```python
from build123d import *

# Parameters (mm, degrees)
SKETCH_1_R      = 40
SKETCH_1_R_2    = 30
EXTRUDE_1_DEPTH = 43
SKETCH_2_R      = 40
EXTRUDE_2_DEPTH = 65
SKETCH_3_R      = 31.5
SKETCH_3_R_2    = 30.5
EXTRUDE_3_DEPTH = 162
FILLET_1_R      = 20
FILLET_2_R      = 20
SKETCH_4_R      = 31.5
SKETCH_4_R_2    = 16
EXTRUDE_4_DEPTH = 1
FILLET_3_R      = 3


with BuildPart() as part:
    # Эскиз1 → Вытянуть1 (new body)
    with BuildSketch(Plane(origin=(0, 0, 0), x_dir=(1, 0, 0), z_dir=(0, 1, 0))):
        with Locations(Location((0, 0, 0), (0, 0, 270))):
            Circle(SKETCH_1_R)
        with Locations(Location((0, 0, 0), (0, 0, 270))):
            Circle(SKETCH_1_R_2, mode=Mode.SUBTRACT)
    extrude(amount=EXTRUDE_1_DEPTH)

    # Эскиз2 → Вытянуть2 (add)
    with BuildSketch(Plane(origin=(0, 43, 0), x_dir=(1, 0, 0), z_dir=(0, 1, 0))):
        with Locations(Location((0, 0, 0), (0, 0, 270))):
            Circle(SKETCH_2_R)
    extrude(amount=EXTRUDE_2_DEPTH)

    # Эскиз3 → Вытянуть3 (add)
    with BuildSketch(Plane(origin=(0, 108, 0), x_dir=(-1, 0, 0), z_dir=(0, 1, 0))):
        with Locations(Location((0, 0, 0), (0, 0, 90))):
            Circle(SKETCH_3_R)
        with Locations(Location((0, 0, 0), (0, 0, 90))):
            Circle(SKETCH_3_R_2, mode=Mode.SUBTRACT)
    extrude(amount=EXTRUDE_3_DEPTH)

    # Скругление1
    # the kernel refuses this fillet: 20 mm, written as the material it adds along each edge
    with BuildSketch(Plane(origin=(0, 108, 0), x_dir=(0, 0, 1), z_dir=(-1, 0, 0))) as fillet_1_piece_1:
        with BuildLine():
            CenterArc((51.5, 16.363068172), FILLET_1_R, 180, 54.900367805)
            Line((31.5, 16.363068172), (31.1, 16.363068172))
            Line((31.1, 16.363068172), (31.1, 0))
            Line((31.1, 0), (31.5, -0.4))
            ThreePointArc((31.5, -0.4), (35.75, -0.4), (39.77, -0.327261363))
            Line((39.77, -0.327261363), (40, 0))
        make_face()
    revolve(axis=Axis((0, 108, 0), (0, 1, 0)))

    # Скругление2
    fillet_2_edges = [part.edges().sort_by_distance(p)[0] for p in [
        (0, 108, -40),
    ]]
    fillet(fillet_2_edges, radius=FILLET_2_R)

    # Эскиз4 → Вытянуть4 (add)
    with BuildSketch(Plane(origin=(0, 270, 0), x_dir=(-1, 0, 0), z_dir=(0, 1, 0))):
        with Locations(Location((0, 0, 0), (0, 0, 270))):
            Circle(SKETCH_4_R)
        with Locations(Location((0, 0, 0), (0, 0, 90))):
            Circle(SKETCH_4_R_2, mode=Mode.SUBTRACT)
    extrude(amount=EXTRUDE_4_DEPTH)

    # Скругление3
    fillet_3_edges = [part.edges().sort_by_distance(p)[0] for p in [
        (0, 271, 31.5),
    ]]
    fillet(fillet_3_edges, radius=FILLET_3_R)


solid = part.part
```
Part model, mm, in its own coordinate system. A direction names the side the tool comes from. Coordinates: 2 decimals unless noted, no trailing zeros. Write each loop counter-clockwise with the first axis right and the second up, starting at its lowest first coordinate (ties: lowest second). Pieces come first, ordered by that corner, then holes.
Item 1: Slice it at B-B (y = 21). Write the cut outline in (x, z).
Item 2: Pin check, flat tips, straight feed: pin 1 (5 mm diameter, centred on x = 30.5, y = 157.5, fed in from -Z); pin 2 (5 mm diameter, centred on y = 67, z = -19.5, fed in from -X); pin 3 (4 mm diameter, centred on y = 216, z = -11, fed in from -X). Stop position of each tip, or through.
Item 3: Slice it at A-A (y = 247). Write the cut outline in (x, z).
Item 4: Probe line 1 (Y direction, x = -12.5, z = -16); line 2 (X direction, y = 28, z = 0); line 3 (X direction, y = 169, z = -1.5). List the from-to ranges inside material, lowest first.
Item 5: Mould opens along X. For faces 1 (the face through (12.015, 49.157, 38.153)), 2 (the face through (14, 271, -12)), 3 (the face through (0, 43, 0)) say: released by +X, released by -X, zero draft, split by the parting line, or undercut.
Item 6: Which spindle directions (+Z, -Z, +X, -X, +Y, -Y) get a long thin tool onto all of the face, cutting with end or side? Do faces 4 (the face through (-15.62, 270.49, -3.47)), 5 (the face through (1.32, 21.2, -29.97)), 6 (the face through (13, 270, -13)). Say none if no direction does.
Results found:
1. outline: circle Ø80 at (0, 0); hole circle Ø60 at (0, 0)
2. pin 1: stops at z = -14.43
2. pin 2: stops at x = -36.21
2. pin 3: stops at x = -30.19
3. outline: circle Ø63 at (0, 0); hole circle Ø61 at (0, 0)
4. line 1: y = 43 to 108, 270 to 271
4. line 2: x = -40 to -30, 30 to 40
4. line 3: x = -31.46 to -30.46, 30.46 to 31.46
5. face 1: split by the parting line
5. face 2: zero draft
5. face 3: undercut
6. face 4: +Y
6. face 5: -Y
6. face 6: none
